For this review, take the finished solid that the model builds, in its own axes (mm). A direction names the side the tool comes from. Round coordinates to 2 decimals unless told otherwise and drop trailing zeros. Write each loop counter-clockwise with the first axis right and the second up, starting at its lowest first coordinate (ties: lowest second). Pieces come first, ordered by that corner, then holes. Notation, with made-up numbers: M -32.75,-29 L -6.75,-29 A22 cw -6.75,-2 Z; hole C 33.25,-26.75 d11. An arc over 180 degrees is marked long. One line per question, with ' | ' between items.
Autodesk Inventor part; units mm, degrees
ref_plane "YZ Plane" through (0, 0, 0) normal (1, 0, 0) x (0, 1, 0)
ref_plane "XZ Plane" through (0, 0, 0) normal (0, 1, 0) x (-1, 0, 0)
ref_plane "XY Plane" through (0, 0, 0) normal (0, 0, 1) x (1, 0, 0)
sketch "Esquisse1" plane through (0, 0, 0) normal (0, 0, 1) x (1, 0, 0)
  line L0 (0, 0) -> (0, 15)
  line L1 (0, 0) -> (80, 0)
  line L2 (80, 0) -> (80, 15)
  arc A0 (0, 15) -> (80, 15) centre (40, 129.2471) ccw
  line L3 (0, 8.2) -> (80, 8.2) construction
  line L4 (40, 0) -> (40, 8.2) construction
  dimension "d0" = 15
  dimension "d1" = 80
  dimension "d28" = 8.2
extrude "Extrusion1" add sketch "Esquisse1" along normal blind 10
sketch "Esquisse2" plane through (0, 0, 10) normal (0, 0, 1) x (1, 0, 0)
  line L0 (0, 0) -> (80, 0)
  line L1 (39, 0) -> (44, 0)
  line L2 (44, 0) -> (44, 8.2)
  line L3 (44, 8.2) -> (39, 8.2)
  line L4 (39, 8.2) -> (39, 0)
  line L5 (0, 15) -> (0, 0)
  line L6 (0, 8.2) -> (80, 8.2) construction
  line L7 (80, 0) -> (80, 15)
  arc A0 (0, 15) -> (80, 15) centre (40, 129.2471) ccw
  line L8 (40, 0) -> (40, 8.2) construction
  dimension "d6" = 5
  dimension "d9" = 80
  dimension "d56" = 4
extrude "Extrusion2" add sketch "Esquisse2" along normal blind 72.9 contours L4 L3 L2 L0
sketch "Esquisse8" plane through (39, 0, 10) normal (-1, 0, 0) x (0, 0, 1)
  circle A0 centre (69.075, 4.1) radius 2
  circle A1 centre (58.975, 4.1) radius 2
  line L0 (0, 8.2) -> (72.9, 8.2)
  line L1 (0, 0) -> (72.9, 0)
  line L2 (72.9, 8.2) -> (72.9, 0)
  point P0 (-10, 0)
  dimension "d45" = 10.1
  dimension "d46" = 4
  dimension "d47" = 4
  dimension "d48" = 8.2
  dimension "d49" = 4.1
  dimension "d50" = 4.1
  dimension "d51" = 3.825
extrude "Extrusion8" cut sketch "Esquisse8" against normal up to surface (5 mm away)
chamfer "Chanfrein1" distance 4 angle 45 2 edges at (39, 4.1, 10) (44, 4.1, 10)
chamfer "Chanfrein2" distance 12 angle 45 2 edges at (0, 0, 5) (80, 0, 5)
fillet "Congé1" radius 2 2 edges at (41.5, 8.2, 82.9) (41.5, 0, 82.9)
equation "\"d47\" = d46"
equation "\"d49\" = 0.5 * d48"
equation "\"d50\" = d49"
properties part number "tete_statique"
Item 1: Insertion check: pin 1 Ø4.5 at (x, y) = (69.5, 10.5) entering from +Z; pin 2 Ø6.5 at (y, z) = (2.5, 44.5) entering from +X; pin 3 Ø4.5 at (y, z) = (4.1, 79.075) entering from -X; pin 4 Ø2 at (x, y) = (54, 10.5) entering from +Z. Each pin has a flat end and moves straight along its axis. Give the tip position at first contact, or say it passes through.
Results:
pin 1: z = 10 | pin 2: x = 44 | pin 3: x = 39 | pin 4: through
Item 2: Take a section at A-A (y = 4.1). Write out the cut boundary in (x, z) (3 decimals), then the cut area to 4 significant figures.
Results:
outline: M 7.9,0 L 72.1,0 L 72.1,10 L 48,10 L 44,14 L 44,66.975 L 39,66.975 L 39,14 L 35,10 L 7.9,10 Z; M 39,70.975 L 44,70.975 L 44,77.075 L 39,77.075 Z; M 39,81.075 L 44,81.075 L 44,82.9 L 39,82.9 Z | area: 982.5 mm2
Item 3: To check wall thickness, follow line 1 along Y through (x, z) = (42, 35); line 2 along X through (y, z) = (6.5, 48); line 3 along Z through (x, y) = (49, 6.5). State the ranges of each line that lie inside material, in increasing order. Write a range as from..to.
Results:
line 1: 0..8.2 | line 2: 39..44 | line 3: 0..10
Item 4: Take a section at C-C (z = 76). Write out the cut boundary in (x, y).
Results:
outline: M 39,0 L 44,0 L 44,8.2 L 39,8.2 Z
Item 5: Machinability: for faces 5 (the face through (41.54, 7.63, 82.3)), 6 (the face through (39, 4, 48)), which of the approach directions +Z, -Z, +X, -X, +Y, -Y give a long, thin tool a straight path to every point of the face, cutting with its end or side? Answer none if there is none.
Results:
face 5: +Z, +X, -X, +Y | face 6: +Z, -X, +Y, -Y
Item 6: Mouldability with a two-part tool opening along Y and no side actions: class faces 1 (the face through (41.46, 5.45, 67.5)), 2 (the face through (6, 6, 5)), 3 (the face through (42, 8.2, 45)), 4 (the face through (44, 4, 48)) as +Y half, -Y half, draft (parallel to the pull), parting line (faces both ways), or undercut.
Results:
face 1: undercut | face 2: -Y half | face 3: +Y half | face 4: draft
Item 7: Take a section at B-B (y = 13.25). Write out the cut boundary in (x, z).
Results:
outline: M 0,0 L 5.4,0 L 5.4,10 L 0,10 Z; M 74.6,0 L 80,0 L 80,10 L 74.6,10 Z
Item 8: Take a section at D-D (x = 29). Write out the cut boundary in (y, z), then the cut area to 3 significant figures.
Results:
outline: M 0,0 L 8.7,0 L 8.7,10 L 0,10 Z | area: 87.0 mm2
